Work out the finished part from the listing and answer in its coordinate system (mm). A direction names the side the tool comes from. Round coordinates to 2 decimals unless told otherwise and drop trailing zeros. Loops run counter-clockwise (first coordinate to the right, second up) from the corner with the lowest first, then second, coordinate; pieces in that order, holes last.
Autodesk Inventor part; units mm, degrees
ref_plane "YZ Plane" through (0, 0, 0) normal (1, 0, 0) x (0, 1, 0)
ref_plane "XZ Plane" through (0, 0, 0) normal (0, 1, 0) x (-1, 0, 0)
ref_plane "XY Plane" through (0, 0, 0) normal (0, 0, 1) x (1, 0, 0)
sketch "Boceto1" plane through (0, 0, 0) normal (0, 1, 0) x (-1, 0, 0)
  line L0 (-54, 30.925) -> (54, 30.925)
  line L1 (54, 30.925) -> (54, -30.925)
  line L2 (54, -30.925) -> (-54, -30.925)
  line L3 (-54, -30.925) -> (-54, 30.925)
  line L4 (-54, 30.925) -> (54, -30.925) construction
  line L5 (54, 30.925) -> (-54, -30.925) construction
  line L6 (54, -30.925) -> (54, -29.075)
  circle A0 centre (-51.1, -27.475) radius 1.6
  circle A1 centre (51.1, -27.475) radius 1.6
  circle A2 centre (51.1, 27.475) radius 1.6
  circle A3 centre (-51.1, 27.475) radius 1.6
  line L7 (54, 30.925) -> (54, 29.075)
  line L8 (-50.7696, -29.075) -> (-51.1, -29.075)
  line L9 (-50.7696, 29.075) -> (-51.1, 29.075)
  line L10 (51.1, 29.075) -> (50.7696, 29.075)
  point P0 (0, 0)
  dimension "d4" = 3.2
  dimension "d6" = 3.2
  dimension "d7" = 3.2
  dimension "d0" = 108
  dimension "d1" = 61.85
  dimension "d5" = 3.2
extrude "Extrusión1" add sketch "Boceto1" along normal blind 1.65
sketch "Boceto2" plane through (0, 1.65, 0) normal (0, 1, 0) x (1, 0, 0)
  line L0 (54, -30.925) -> (54, 30.925)
  line L1 (54, 30.925) -> (-54, 30.925)
  line L2 (-54, 30.925) -> (-54, -30.925)
  line L3 (-54, -30.925) -> (54, -30.925)
  circle A0 centre (51.1, 27.475) radius 1.6
  circle A1 centre (-51.1, 27.475) radius 1.6
  circle A2 centre (-51.1, -27.475) radius 1.6
  circle A3 centre (51.1, -27.475) radius 1.6
  line L4 (54, 30.925) -> (54, 5.075)
  line L5 (54, -30.925) -> (54, 30.925)
  line L6 (54, 5.075) -> (53.25, 5.075)
  line L7 (53.25, 5.075) -> (50.71, 5.075)
  line L8 (50.71, 5.075) -> (50.71, -5.085)
  line L9 (50.71, -5.085) -> (53.25, -5.085)
  line L10 (53.25, -5.085) -> (53.25, 5.075)
  line L11 (51.98, 5.075) -> (51.98, -5.085)
  line L12 (51.98, 5.075) -> (51.98, 3.805)
  line L13 (51.98, 3.805) -> (51.98, 1.265)
  line L14 (51.98, 1.265) -> (51.98, -1.275)
  line L15 (51.98, -1.275) -> (51.98, -3.815)
  circle A4 centre (51.98, 3.805) radius 0.5
  circle A5 centre (51.98, 1.265) radius 0.5
  circle A6 centre (51.98, -1.275) radius 0.5
  circle A7 centre (51.98, -3.815) radius 0.5
  line L16 (-54, 30.925) -> (-53.25, 30.925)
  line L17 (54, 30.925) -> (-54, 30.925)
  line L18 (-53.25, 30.925) -> (-53.25, 17.675)
  line L19 (-53.25, 17.675) -> (-50.71, 17.675)
  line L20 (-50.71, 17.675) -> (-50.71, -17.885)
  line L21 (-50.71, -17.885) -> (-53.25, -17.885)
  line L22 (-53.25, -17.885) -> (-53.25, 17.675)
  line L23 (-51.98, 17.675) -> (-51.98, 16.405)
  circle A8 centre (-51.98, 16.405) radius 0.5
  line L24 (-51.98, 16.405) -> (-51.98, 13.851)
  line L25 (-51.98, 15.121) -> (-51.98, 13.851)
  circle A9 centre (-51.98, 13.851) radius 0.5
  line L26 (-51.98, 13.851) -> (-51.98, 11.297)
  line L27 (-51.98, 12.567) -> (-51.98, 11.297)
  circle A10 centre (-51.98, 11.297) radius 0.5
  line L28 (-51.98, 11.297) -> (-51.98, 8.743)
  line L29 (-51.98, 8.743) -> (-51.98, 6.189)
  circle A11 centre (-51.98, 8.743) radius 0.5
  line L30 (-51.98, 6.189) -> (-51.98, 3.635)
  circle A12 centre (-51.98, 6.189) radius 0.5
  line L31 (-51.98, 3.635) -> (-51.98, 1.081)
  circle A13 centre (-51.98, 3.635) radius 0.5
  line L32 (-51.98, 1.081) -> (-51.98, -1.473)
  circle A14 centre (-51.98, 1.081) radius 0.5
  line L33 (-51.98, -1.473) -> (-51.98, -4.027)
  circle A15 centre (-51.98, -1.473) radius 0.5
  line L34 (-51.98, -4.027) -> (-51.98, -6.581)
  circle A16 centre (-51.98, -4.027) radius 0.5
  line L35 (-51.98, -6.581) -> (-51.98, -9.135)
  circle A17 centre (-51.98, -6.581) radius 0.5
  line L36 (-51.98, -9.135) -> (-51.98, -11.689)
  circle A18 centre (-51.98, -9.135) radius 0.5
  line L37 (-51.98, -11.689) -> (-51.98, -14.243)
  circle A19 centre (-51.98, -11.689) radius 0.5
  line L38 (-51.98, -14.243) -> (-51.98, -16.797)
  circle A20 centre (-51.98, -14.243) radius 0.5
  line L39 (-51.98, -16.797) -> (-51.98, -19.351)
  circle A21 centre (-51.98, -16.797) radius 0.5
  point P0 (0, 0)
  dimension "d11" = 25.85
  dimension "d12" = 0.75
  dimension "d13" = 2.54
  dimension "d14" = 10.16
  dimension "d15" = 1.27
  dimension "d16" = 2.54
  dimension "d17" = 2.54
  dimension "d18" = 2.54
  dimension "d19" = 1
  dimension "d20" = 1
  dimension "d21" = 1
  dimension "d22" = 1
  dimension "d30" = 0.75
  dimension "d31" = 13.25
  dimension "d32" = 2.54
  dimension "d33" = 35.56
  dimension "d34" = 1.27
  dimension "d35" = 1
  dimension "d36" = 2.554
  dimension "d37" = 1.27
  dimension "d38" = 1
  dimension "d39" = 2.554
  dimension "d40" = 1.27
  dimension "d41" = 1
  dimension "d42" = 2.554
  dimension "d43" = 1
  dimension "d44" = 2.554
  dimension "d45" = 1
  dimension "d46" = 2.554
  dimension "d47" = 1
  dimension "d48" = 2.554
  dimension "d49" = 1
  dimension "d50" = 2.554
  dimension "d51" = 1
  dimension "d52" = 2.554
  dimension "d53" = 1
  dimension "d54" = 2.554
  dimension "d55" = 1
  dimension "d56" = 2.554
  dimension "d57" = 1
  dimension "d58" = 2.554
  dimension "d59" = 1
  dimension "d60" = 2.554
  dimension "d61" = 1
  dimension "d62" = 2.554
  dimension "d63" = 1
  dimension "d64" = 2.554
hole "Agujero1" at (51.98, 1.65, -3.805) at (51.98, 1.65, -1.265) at (51.98, 1.65, 1.275) at (51.98, 1.65, 3.815) at (-51.98, 1.65, -16.405) at (-51.98, 1.65, -13.851) at (-51.98, 1.65, -11.297) at (-51.98, 1.65, -8.743) at (-51.98, 1.65, -6.189) at (-51.98, 1.65, -3.635) at (-51.98, 1.65, -1.081) at (-51.98, 1.65, 1.473) at (-51.98, 1.65, 4.027) at (-51.98, 1.65, 6.581) at (-51.98, 1.65, 9.135) at (-51.98, 1.65, 11.689) at (-51.98, 1.65, 14.243) at (-51.98, 1.65, 16.797) direction (0, -1, 0) diameter 1 end through all
sketch "Boceto3" plane through (0, 1.65, 0) normal (0, 1, 0) x (1, 0, 0)
  circle A0 centre (-51.98, -16.797) radius 0.5
  circle A1 centre (-51.98, -14.243) radius 0.5
  circle A2 centre (-51.98, -11.689) radius 0.5
  circle A3 centre (-51.98, -9.135) radius 0.5
  circle A4 centre (-51.98, -6.581) radius 0.5
  circle A5 centre (-51.98, -4.027) radius 0.5
  circle A6 centre (-51.98, -1.473) radius 0.5
  circle A7 centre (-51.98, 1.081) radius 0.5
  circle A8 centre (-51.98, 3.635) radius 0.5
  circle A9 centre (-51.98, 6.189) radius 0.5
  circle A10 centre (-51.98, 8.743) radius 0.5
  circle A11 centre (-51.98, 11.297) radius 0.5
  circle A12 centre (-51.98, 13.851) radius 0.5
  circle A13 centre (-51.98, 16.405) radius 0.5
  circle A14 centre (51.98, -3.815) radius 0.5
  circle A15 centre (51.98, -1.275) radius 0.5
  circle A16 centre (51.98, 1.265) radius 0.5
  circle A17 centre (51.98, 3.805) radius 0.5
  line L0 (54, -30.925) -> (54, 30.925)
  line L1 (54, 30.925) -> (-54, 30.925)
  line L2 (-54, 30.925) -> (-54, -30.925)
  line L3 (-54, -30.925) -> (54, -30.925)
  circle A18 centre (51.1, 27.475) radius 1.6
  circle A19 centre (-51.1, 27.475) radius 1.6
  circle A20 centre (-51.1, -27.475) radius 1.6
  circle A21 centre (51.1, -27.475) radius 1.6
  line L4 (-51.98, 17.675) -> (-50.71, 17.675)
  line L5 (-50.71, 17.675) -> (-53.25, 17.675)
  line L6 (-53.25, 17.675) -> (-53.25, -17.885)
  line L7 (-53.25, -17.885) -> (-50.71, -17.885)
  line L8 (-50.71, -17.885) -> (-50.71, 17.675)
  line L9 (-53.25, 17.675) -> (-53.25, 15.135)
  line L10 (-53.25, 15.135) -> (-50.71, 15.135)
  line L11 (51.98, 5.075) -> (53.25, 5.075)
  line L12 (53.25, 5.075) -> (50.71, 5.075)
  line L13 (50.71, 5.075) -> (50.71, -5.085)
  line L14 (50.71, -5.085) -> (53.25, -5.085)
  line L15 (53.25, -5.085) -> (53.25, 5.075)
  line L16 (50.71, -5.085) -> (50.71, -4.818)
  line L17 (50.71, 5.075) -> (50.71, 2.535)
  line L18 (50.71, 2.535) -> (53.25, 2.535)
  line L19 (54, 30.925) -> (-54, 30.925)
  line L20 (-47.6, 30.225) -> (47, 30.225)
  line L21 (47, 30.225) -> (47, -30.225)
  line L22 (47, -30.225) -> (-47.6, -30.225)
  line L23 (-47.6, -30.225) -> (-47.6, 30.225)
  point P0 (0, 0)
sketch "Boceto4" plane through (0, 1.65, 0) normal (0, 1, 0) x (1, 0, 0)
  line L0 (-47.6, -30.225) -> (-47.6, 30.225)
  line L1 (47, 30.225) -> (47, -30.225)
  line L2 (-47.6, 30.225) -> (47, 30.225)
  line L3 (47, -30.225) -> (-47.6, -30.225)
  point P0 (0, 0)
extrude "Extrusión2" add sketch "Boceto4" along normal blind 4.15
sketch "Boceto5" plane through (0, 0, 0) normal (0, -1, 0) x (1, 0, 0)
  circle A0 centre (-51.98, 16.797) radius 0.5
  circle A1 centre (-51.98, 14.243) radius 0.5
  circle A2 centre (-51.98, 11.689) radius 0.5
  circle A3 centre (-51.98, 9.135) radius 0.5
  circle A4 centre (-51.98, 6.581) radius 0.5
  circle A5 centre (-51.98, 4.027) radius 0.5
  circle A6 centre (-51.98, 1.473) radius 0.5
  circle A7 centre (-51.98, -1.081) radius 0.5
  circle A8 centre (-51.98, -3.635) radius 0.5
  circle A9 centre (-51.98, -6.189) radius 0.5
  circle A10 centre (-51.98, -8.743) radius 0.5
  circle A11 centre (-51.98, -11.297) radius 0.5
  circle A12 centre (-51.98, -13.851) radius 0.5
  circle A13 centre (-51.98, -16.405) radius 0.5
  circle A14 centre (51.98, 3.815) radius 0.5
  circle A15 centre (51.98, 1.275) radius 0.5
  circle A16 centre (51.98, -1.265) radius 0.5
  circle A17 centre (51.98, -3.805) radius 0.5
  line L0 (54, 30.925) -> (54, -30.925)
  line L1 (-54, 30.925) -> (54, 30.925)
  line L2 (-54, -30.925) -> (-54, 30.925)
  line L3 (54, -30.925) -> (-54, -30.925)
  circle A18 centre (51.1, -27.475) radius 1.6
  circle A19 centre (-51.1, -27.475) radius 1.6
  circle A20 centre (-51.1, 27.475) radius 1.6
  circle A21 centre (51.1, 27.475) radius 1.6
  line L4 (54, -30.925) -> (45.6, -30.925)
  line L5 (45.6, -30.925) -> (19.1, -30.925)
  line L6 (19.1, -30.925) -> (19.1, -10.525)
  line L7 (19.1, -10.525) -> (45.6, -10.525)
  line L8 (45.6, -10.525) -> (45.6, -30.925)
  line L9 (45.6, -30.925) -> (45.6, -29.925)
  line L10 (45.6, -29.925) -> (19.1, -29.925)
  point P0 (0, 0)
  dimension "d81" = 8.4
  dimension "d82" = 26.5
  dimension "d83" = 20.4
  dimension "d86" = 1
extrude "Extrusión3" add sketch "Boceto5" along normal blind 3 contours L10 L6 L7 L8
properties part number "ILI9488"
1. Consider probe 1 along Y at (x, z) = (-41, -22); probe 2 along X at (y, z) = (3.5, 8); probe 3 along X at (y, z) = (-2.25, -22). Determine where each line is inside the solid, lowest interval first.
Answer key:
probe 1: y = 0 to 5.8
probe 2: x = -47.6 to 47
probe 3: x = 19.1 to 45.6
2. Which of the six approach directions +Z, -Z, +X, -X, +Y, -Y give full straight-line access (tool end or side, diameter ignored) to faces 4 (the face through (0, 4, 30.225)), 5 (the face through (32, -1, -10.525)), 6 (the face through (-1, 4, -30.225)), 7 (the face through (45.6, -1, -20)), 8 (the face through (33, -1, -29.925))?
Answer key:
face 4: +Z, +X, -X, +Y
face 5: +Z, +X, -X, -Y
face 6: -Z, +X, -X, +Y
face 7: +Z, -Z, +X, -Y
face 8: -Z, +X, -X, -Y
3. Find section B-B (z = -22.5). Write down the section's boundary in (x, y).
Answer key:
outline: (-54, 0) - (19.1, 0) - (19.1, -3) - (45.6, -3) - (45.6, 0) - (54, 0) - (54, 1.65) - (47, 1.65) - (47, 5.8) - (-47.6, 5.8) - (-47.6, 1.65) - (-54, 1.65) - close
4. Determine the mould class of faces 1 (the face through (-47.6, 4, 0)), 2 (the face through (47, 4, 0)), 3 (the face through (49.574, 0.813, -27.956)) for opening direction X: +X half, -X half, draft (parallel to the pull), parting line (faces both ways), or undercut.
Answer key:
face 1: -X half
face 2: +X half
face 3: undercut
5. Find section D-D (y = -1.75). Write down the section's boundary in (x, z) (3 decimals).
Answer key:
outline: (19.1, -29.925) - (45.6, -29.925) - (45.6, -10.525) - (19.1, -10.525) - close
6. Find section C-C (y = 3.75). Write down the section's boundary in (x, z) (3 decimals).
Answer key:
outline: (-47.6, -30.225) - (47, -30.225) - (47, 30.225) - (-47.6, 30.225) - close
7. Given pin 1 (2 mm diameter, centred on y = 4.5, z = -11, fed in from +X); pin 2 (5 mm diameter, centred on x = -51.1, z = 27.475, fed in from +Y); pin 3 (3.5 mm diameter, centred on x = 30.5, y = -2, fed in from -Z) (3 decimals), each flat-ended and moving along its own axis, determine where each tip first touches the part or whether it passes through.
Answer key:
pin 1: stops at x = 47
pin 2: stops at y = 1.65
pin 3: stops at z = -29.925
8. Find section A-A (x = -13). Write down the section's boundary in (y, z) (3 decimals).
Answer key:
outline: (0, -30.925) - (1.65, -30.925) - (1.65, -30.225) - (5.8, -30.225) - (5.8, 30.225) - (1.65, 30.225) - (1.65, 30.925) - (0, 30.925) - close
